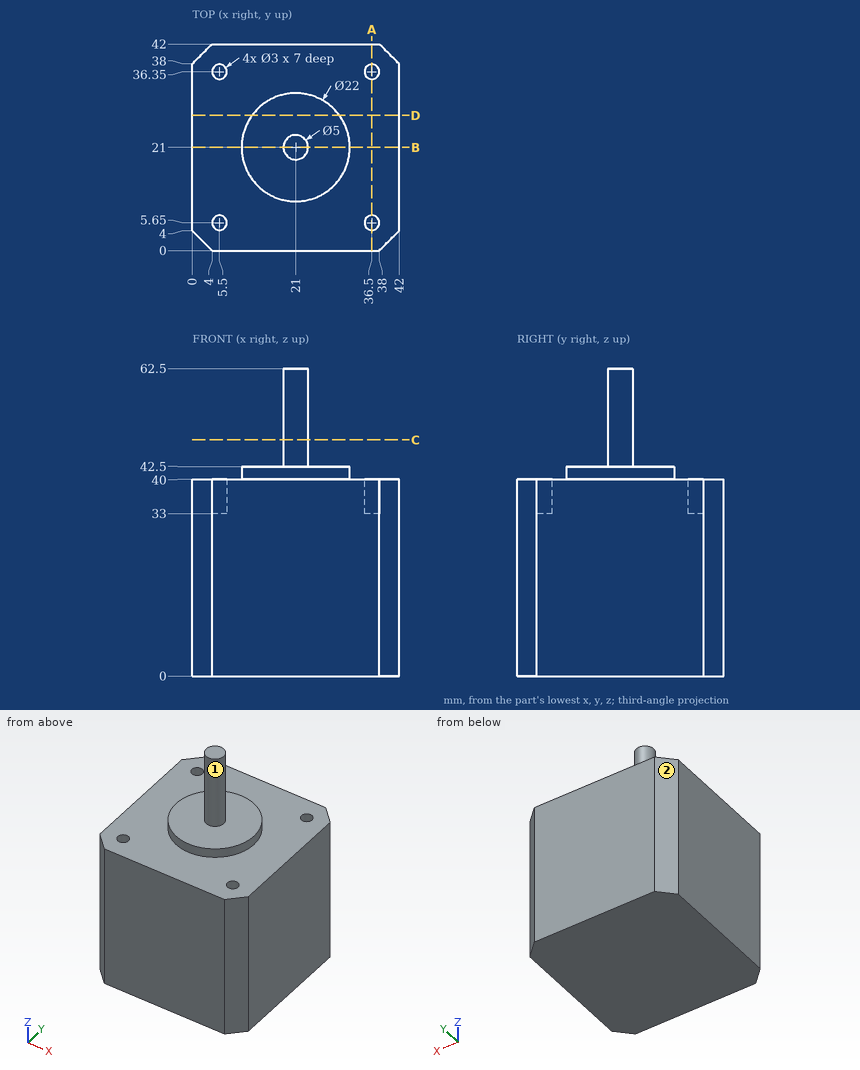
Answer from the drawing. Dimensions are ordinates in mm from the lowest x, y and z of the part. A direction names the side the tool comes from. Coordinates: 2 decimals unless noted, no trailing zeros. Loops run counter-clockwise (first coordinate to the right, second up) from the corner with the lowest first, then second, coordinate; pieces in that order, holes last.
Q1. The part is cut by section A-A on x = 36.5. Write down the section's boundary in (y, z).
Q2. The part is cut by section B-B on y = 21. Write down the section's boundary in (x, z), and give its area (4 significant figures).
Q3. Each of these flat-tipped pins is pushed along its axis until it touches: pin 1 Ø3.5 at (x, y) = (36, 36.5) entering from +Z; pin 2 Ø1.8 at (x, y) = (5.5, 5.65) entering from -Z; pin 3 Ø6 at (x, y) = (17, 13) entering from +Z; pin 4 Ø0.9 at (x, y) = (6, 36.5) entering from +Z. Where does it stop, or does it pass through?
Q4. The part is cut by section C-C on z = 48. Write down the section's boundary in (x, y).
Q5. Consider probe 1 along Y at (x, z) = (5.5, 37); probe 2 along Z at (x, y) = (6, 14); probe 3 along Z at (x, y) = (18.5, 30). Determine where each line is inside the solid, lowest interval first.
Q6. Which of the six approach directions +Z, -Z, +X, -X, +Y, -Y give full straight-line access (tool end or side, diameter ignored) to the marked faces 1 and 2?
Q7. The part is cut by section D-D on y = 27.5. Write down the section's boundary in (x, z) (1 decimal).
Results below:
1. outline: (0, 0) - (42, 0) - (42, 40) - (37.85, 40) - (37.85, 33) - (34.85, 33) - (34.85, 40) - (7.15, 40) - (7.15, 33) - (4.15, 33) - (4.15, 40) - (0, 40) - close
2. outline: (0, 0) - (42, 0) - (42, 40) - (32, 40) - (32, 42.5) - (23.5, 42.5) - (23.5, 62.5) - (18.5, 62.5) - (18.5, 42.5) - (10, 42.5) - (10, 40) - (0, 40) - close
2. area: 1,835 mm2
3. pin 1: stops at z = 40
3. pin 2: stops at z = 0
3. pin 3: stops at z = 42.5
3. pin 4: stops at z = 33
4. outline: circle Ø5 at (21, 21)
5. probe 1: y = 0 to 4.15, 7.15 to 34.85, 37.85 to 42
5. probe 2: z = 0 to 40
5. probe 3: z = 0 to 42.5
6. face 1: +Z
6. face 2: +Z, -Z, -X, +Y
7. outline: (0, 0) - (42, 0) - (42, 40) - (29.9, 40) - (29.9, 42.5) - (12.1, 42.5) - (12.1, 40) - (0, 40) - close
